Source: CAD feature listing. Evaluate the final solid. Frame: model axes, mm. Face numbers are marked on the shaded views. A direction names the side the tool comes from. Round coordinates to 2 decimals unless told otherwise and drop trailing zeros. Write each loop counter-clockwise with the first axis right and the second up, starting at its lowest first coordinate (ties: lowest second). Pieces come first, ordered by that corner, then holes. Notation, with made-up numbers: M 48.5,-33.75 L 86.5,-33.75 A17 cw 86.5,-6.75 Z; hole C 36.5,3 d6. An arc over 180 degrees is marked long. Use a Markdown table: item, result.
```python
from build123d import *

# Parameters (mm, degrees)
BOSS_EXTRUDE6_DEPTH = 7.5
BOSS_EXTRUDE7_DEPTH = 7.5


with BuildPart() as part:
    # Sketch1 → Boss-Extrude6 (new body)
    with BuildSketch(Plane(origin=(0, 0, 0), x_dir=(1, 0, 0), z_dir=(0, 1, 0))):
        Polygon((0, -7.5), (125, -7.5), (125, 0), (150, 54), (150, 96), (125, 150), (125, 157.5), (0, 157.5), (0, 150), (-30, 90), (-30, 60), (0, 0), align=None)
        with BuildLine():
            Line((134.5, 55.5), (134.5, 94.5))
            ThreePointArc((134.5, 94.5), (137.5, 97.5), (140.5, 94.5))
            Line((140.5, 94.5), (140.5, 55.5))
            ThreePointArc((140.5, 55.5), (137.5, 52.5), (134.5, 55.5))
        make_face(mode=Mode.SUBTRACT)
        with BuildLine():
            Line((-17, 55.5), (-17, 94.5))
            ThreePointArc((-17, 94.5), (-14, 97.5), (-11, 94.5))
            Line((-11, 94.5), (-11, 55.5))
            ThreePointArc((-11, 55.5), (-14, 52.5), (-17, 55.5))
        make_face(mode=Mode.SUBTRACT)
        with BuildLine():
            Line((59.5, 11), (59.5, 50))
            ThreePointArc((59.5, 50), (62.5, 53), (65.5, 50))
            Line((65.5, 50), (65.5, 11))
            ThreePointArc((65.5, 11), (62.5, 8), (59.5, 11))
        make_face(mode=Mode.SUBTRACT)
        with BuildLine():
            Line((65.5, 138.705746838), (65.5, 99.705746838))
            ThreePointArc((65.5, 99.705746838), (62.5, 96.705746838), (59.5, 99.705746838))
            Line((59.5, 99.705746838), (59.5, 138.705746838))
            ThreePointArc((59.5, 138.705746838), (62.5, 141.705746839), (65.5, 138.705746838))
        make_face(mode=Mode.SUBTRACT)
    extrude(amount=BOSS_EXTRUDE6_DEPTH)

    # Sketch2 → Boss-Extrude7 (add)
    with BuildSketch(Plane.XY):
        with BuildLine():
            Line((0, 0), (0, 118))
            ThreePointArc((0, 118), (0.585786438, 119.414213562), (2, 120))
            Line((2, 120), (47.812758192, 120))
            ThreePointArc((47.812758192, 120), (49.226971755, 119.414213562), (49.812758192, 118))
            Line((49.812758192, 118), (49.812758192, 80))
            ThreePointArc((49.812758192, 80), (52.74169038, 72.928932188), (59.812758192, 70))
            Line((59.812758192, 70), (64.812758192, 70))
            ThreePointArc((64.812758192, 70), (71.883826004, 72.928932188), (74.812758192, 80))
            Line((74.812758192, 80), (74.812758192, 118))
            ThreePointArc((74.812758192, 118), (75.39854463, 119.414213562), (76.812758192, 120))
            Line((76.812758192, 120), (122.812758192, 120))
            ThreePointArc((122.812758192, 120), (124.226971755, 119.414213562), (124.812758192, 118))
            Line((124.812758192, 118), (124.812758192, 0))
            Line((124.812758192, 0), (0, 0))
        make_face()
        with BuildLine():
            Line((36.312758192, 88.190430343), (36.312758192, 109.809569657))
            ThreePointArc((36.312758192, 109.809569657), (39.812758192, 113.309569657), (43.312758192, 109.809569657))
            Line((43.312758192, 109.809569657), (43.312758192, 88.190430343))
            ThreePointArc((43.312758192, 88.190430343), (39.812758192, 84.690430343), (36.312758192, 88.190430343))
        make_face(mode=Mode.SUBTRACT)
        with BuildLine():
            Line((88.312758192, 88.190430343), (88.312758192, 109.809569657))
            ThreePointArc((88.312758192, 109.809569657), (84.812758192, 113.309569657), (81.312758192, 109.809569657))
            Line((81.312758192, 109.809569657), (81.312758192, 88.190430343))
            ThreePointArc((81.312758192, 88.190430343), (84.812758192, 84.690430343), (88.312758192, 88.190430343))
        make_face(mode=Mode.SUBTRACT)
    boss_extrude7 = extrude(amount=BOSS_EXTRUDE7_DEPTH)

    # Mirror1: Boss-Extrude7 across plane
    add(boss_extrude7.mirror(Plane(origin=(0, 0, -75), x_dir=(1, 0, 0), z_dir=(0, 0, -1))))


solid = part.part
```
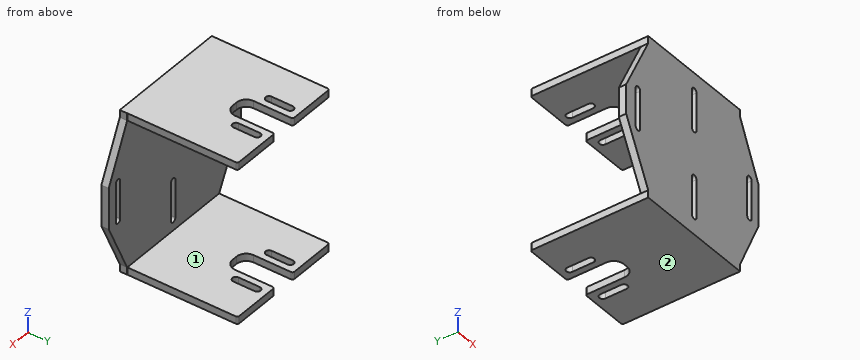
Q1. Section B-B on x = -14. Return loops of the section in (y, z).
Results are:
| item | result |
|---|---|
| outline | M 0,-122 L 7.5,-122 L 7.5,-97.5 L 0,-97.5 Z; M 0,-52.5 L 7.5,-52.5 L 7.5,-28 L 0,-28 Z |
Q2. Line query: L1, parallel to Z at x = 7, y = 60; L2, parallel to Y at x = 118, z = -17. Output: solid intervals per line, ascending.
Results are:
| item | result |
|---|---|
| L1 | -157.5 to -150, 0 to 7.5 |
| L2 | 0 to 7.5 |
Q3. First-contact query: pin 1 Ø2 at (y, z) = (91.5, -153.5) entering from -X; pin 2 Ø5 at (x, z) = (10, -83) entering from +Y; pin 3 Ø2 at (y, z) = (4.5, -29.5) entering from +X. Flat tips, straight axial feed; report the tip coordinate or a pass-through.
Results are:
| item | result |
|---|---|
| pin 1 | x = 0 |
| pin 2 | y = 7.5 |
| pin 3 | x = 139.12 |
Q4. Reachability of the marked faces 1 and 2 from +Z, -Z, +X, -X, +Y, -Y: full face, straight path, thin tool, end or side. Return the list, or none.
Results are:
| item | result |
|---|---|
| face 1 | +X, -X, +Y |
| face 2 | -Z, +X, -X, +Y, -Y |
Q5. Section D-D on x = 30. Return loops of the section in (y, z), plus the area to 4 significant figures.
Results are:
| item | result |
|---|---|
| outline | M 0,-157.5 L 120,-157.5 L 120,-150 L 7.5,-150 L 7.5,0 L 120,0 L 120,7.5 L 0,7.5 Z |
| area | 2,925 mm^2 |
Q6. Section C-C on x = 62.5. Return loops of the section in (y, z).
Results are:
| item | result |
|---|---|
| outline | M 0,-157.5 L 70,-157.5 L 70,-150 L 7.5,-150 L 7.5,-141.71 L 0,-141.71 Z; M 0,-96.71 L 7.5,-96.71 L 7.5,-53 L 0,-53 Z; M 0,-8 L 7.5,-8 L 7.5,0 L 70,0 L 70,7.5 L 0,7.5 Z |
Q7. Section A-A on y = 48.5. Return loops of the section in (x, z).
Results are:
| item | result |
|---|---|
| outline | M 0,-157.5 L 124.81,-157.5 L 124.81,-150 L 0,-150 Z; M 0,0 L 124.81,0 L 124.81,7.5 L 0,7.5 Z |
